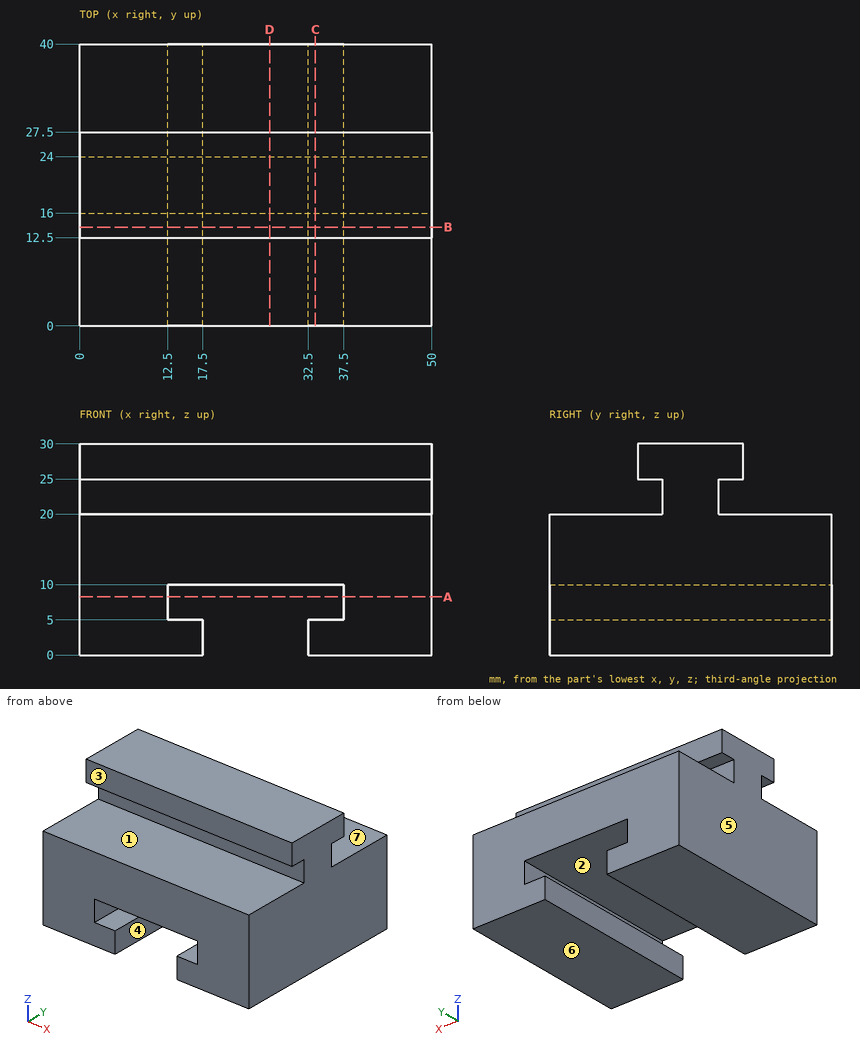
Here's the drawing with two shaded views (mm, measured from the low corner). I have some questions. A direction names the side the tool comes from. Coordinates: 2 decimals unless noted, no trailing zeros. Loops run counter-clockwise (first coordinate to the right, second up) from the corner with the lowest first, then second, coordinate; pieces in that order, holes last. Notation, with made-up numbers: (66, -15.5) - (94, -15.5) arc R36 cw to (94, 18.5) - close; hole circle Ø2 at (44, 77). An arc over 180 degrees is marked (long way). Answer as CSV lines item,"result". Start each with the question number.
1) Suppose I cut it at C-C (x = 33.5). Please give me the cut outline in (y, z), plus the area to 3 significant figures.
2) Thinking about a two-plate mould opening in Z: for the marked faces 5, 6 and 7, which applies, pulls with the +Z half, pulls with the -Z half, needs draft (parallel to the pull), parting line crosses it, or undercut?
3) Suppose I cut it at D-D (x = 27). Please give me the cut outline in (y, z), plus the area to 3 significant figures.
4) Suppose I cut it at B-B (y = 14). Please give me the cut outline in (x, z).
5) I need wall thicknesses on line 1 (Z direction, x = 24.5, y = 25); line 2 (X direction, y = 6.5, z = 1.5); line 3 (X direction, y = 14, z = 8). Which ranges of each line are inside material? Lowest first, please. Write a range as from..to.
6) Which directions (+Z, -Z, +X, -X, +Y, -Y) give clear straight access to the entire face, cutting with the end or side of a thin tool? Please do the marked faces 1, 2, 3 and 4.
7) Suppose I cut it at A-A (z = 8.25). Please give me the cut outline in (x, y), plus the area to 3 significant figures.
8) For pin 1 (8 mm diameter, centred on x = 31.5, y = 7, fed in from +Z); pin 2 (2.5 mm diameter, centred on x = 19, z = 23, fed in from -Y); pin 3 (1.8 mm diameter, centred on x = 21.5, y = 25.5, fed in from -Z); pin 4 (1 mm diameter, centred on y = 27.5, z = 22, fed in from -X), each with a flat end and sliding along its axis, tell me the tip position at first contact or that it passes through.
Check result:
1,outline,"(0, 0) - (40, 0) - (40, 5) - (0, 5) - close; (0, 10) - (40, 10) - (40, 20) - (24, 20) - (24, 25) - (27.5, 25) - (27.5, 30) - (12.5, 30) - (12.5, 25) - (16, 25) - (16, 20) - (0, 20) - close"
1,area,"715 mm²"
2,face 5,"needs draft"
2,face 6,"pulls with the -Z half"
2,face 7,"undercut"
3,outline,"(0, 10) - (40, 10) - (40, 20) - (24, 20) - (24, 25) - (27.5, 25) - (27.5, 30) - (12.5, 30) - (12.5, 25) - (16, 25) - (16, 20) - (0, 20) - close"
3,area,"515 mm²"
4,outline,"(0, 0) - (17.5, 0) - (17.5, 5) - (12.5, 5) - (12.5, 10) - (37.5, 10) - (37.5, 5) - (32.5, 5) - (32.5, 0) - (50, 0) - (50, 20) - (0, 20) - close; (0, 25) - (50, 25) - (50, 30) - (0, 30) - close"
5,line 1,"z = 10..20, 25..30"
5,line 2,"x = 0..17.5, 32.5..50"
5,line 3,"x = 0..12.5, 37.5..50"
6,face 1,"+X, -X, -Y"
6,face 2,"+Y, -Y"
6,face 3,"+Z, +X, -X, -Y"
6,face 4,"-Z, +Y, -Y"
7,outline,"(0, 0) - (12.5, 0) - (12.5, 40) - (0, 40) - close; (37.5, 0) - (50, 0) - (50, 40) - (37.5, 40) - close"
7,area,"1,000 mm²"
8,pin 1,"stops at z = 20"
8,pin 2,"stops at y = 16"
8,pin 3,"stops at z = 10"
8,pin 4,"passes through"
